from build123d import *

# Parameters (mm, degrees)
SKETCH_1_W          = 24
SKETCH_1_H          = 12
EXTRUDE_1_DEPTH     = 12
SKETCH_2_R          = 1
EXTRUDE_2_DEPTH     = 1.8
SKETCH_3_W          = 24
SKETCH_3_H          = 12
EXTRUDE_3_DEPTH     = 4
EXTRUDE_4_DEPTH     = 4
SKETCH_5_R          = 2
EXTRUDE_5_DEPTH     = 3.5
EXTRUDE_6_DEPTH     = 3
CUT_EXTRUDE_1_DEPTH = 12


with BuildPart() as part:
    # Эскиз1 → Бобышка-Вытянуть1 (new body)
    with BuildSketch(Plane.XY):
        Rectangle(SKETCH_1_W, SKETCH_1_H)
    extrude(amount=EXTRUDE_1_DEPTH)

    # Эскиз2 → Бобышка-Вытянуть2 (add)
    with BuildSketch(Plane(origin=(0, 0, 0), x_dir=(-1, 0, 0), z_dir=(0, 0, -1))):
        with BuildLine():
            Line((12, 6), (15, 6))
            ThreePointArc((15, 6), (15.707106781, 5.707106781), (16, 5))
            Line((16, 5), (16, -5))
            ThreePointArc((16, -5), (15.707106781, -5.707106781), (15, -6))
            Line((15, -6), (12, -6))
            Line((12, -6), (-12, -6))
            Line((-12, -6), (-15, -6))
            ThreePointArc((-15, -6), (-15.707106781, -5.707106781), (-16, -5))
            Line((-16, -5), (-16, 5))
            ThreePointArc((-16, 5), (-15.707106781, 5.707106781), (-15, 6))
            Line((-15, 6), (-12, 6))
            Line((-12, 6), (12, 6))
        make_face()
        with Locations((14, 0)):
            Circle(SKETCH_2_R, mode=Mode.SUBTRACT)
        with Locations((-14, 0)):
            Circle(SKETCH_2_R, mode=Mode.SUBTRACT)
    extrude(amount=EXTRUDE_2_DEPTH)

    # Эскиз3 → Бобышка-Вытянуть3 (add)
    with BuildSketch(Plane(origin=(0, 0, -1.8), x_dir=(-1, 0, 0), z_dir=(0, 0, -1))):
        Rectangle(SKETCH_3_W, SKETCH_3_H)
    extrude(amount=EXTRUDE_3_DEPTH)

    # Эскиз4 → Бобышка-Вытянуть4 (add)
    with BuildSketch(Plane(origin=(0, 0, -5.8), x_dir=(-1, 0, 0), z_dir=(0, 0, -1))):
        with BuildLine():
            ThreePointArc((0.75, 2.90473751), (12, 0), (0.75, -2.90473751))
            ThreePointArc((0.75, -2.90473751), (-3, 0), (0.75, 2.90473751))
        make_face()
    extrude(amount=EXTRUDE_4_DEPTH)

    # Эскиз5 → Бобышка-Вытянуть5 (add)
    with BuildSketch(Plane(origin=(0, 0, -9.8), x_dir=(-1, 0, 0), z_dir=(0, 0, -1))):
        with Locations((6, 0)):
            Circle(SKETCH_5_R)
    extrude(amount=EXTRUDE_5_DEPTH)

    # Эскиз6 → Бобышка-Вытянуть6 (add)
    with BuildSketch(Plane.XY.offset(12)):
        Polygon((12, -6), (12, 6), (-10, 6), (-10, 4), (-12, 4), (-12, -4), (-10, -4), (-10, -6), align=None)
    extrude(amount=EXTRUDE_6_DEPTH)

    # Эскиз8 → Вырез-Вытянуть1 (cut)
    with BuildSketch(Plane(origin=(0, 6, 0), x_dir=(1, 0, 0), z_dir=(0, 1, 0))):
        Polygon((-7, -15), (-12, -12), (-12, -15), align=None)
    extrude(amount=-CUT_EXTRUDE_1_DEPTH, mode=Mode.SUBTRACT)


solid = part.part
Verification items for the finished model (mm, model axes). A direction names the side the tool comes from. Round coordinates to 2 decimals unless told otherwise and drop trailing zeros. Order: outer loops, then holes, each group sorted by start corner. A loop starts at its lowest first (then second) coordinate and runs counter-clockwise, first axis right, second up. Notation, with made-up numbers: (61.5, -6) -> (72.5, -6) arc R16 ccw to (72.5, -1) -> close; hole circle Ø1 at (78, -33.75). An arc over 180 degrees is marked (long way). Put each result on its own line as item: value.
1) Section check C-C (z = -10.25). Record the cut outline in (x, y).
Final values:
outline: circle Ø4 at (-6, 0)
2) Section check D-D (z = 9). Record the cut outline in (x, y).
Final values:
outline: (-12, -6) -> (12, -6) -> (12, 6) -> (-12, 6) -> close
3) Set-up check for faces 1 (the flat face through (-3, 0, -9.8)), 2 (the flat face through (-10, 5, 13)), 3 (the flat face through (15.3, 0.1, -1.8)): record each of +Z, -Z, +X, -X, +Y, -Y from which the full face is reachable in a straight line by a thin tool's end or side.
Final values:
face 1: -Z
face 2: +Z, -X, +Y
face 3: -Z, +X, +Y, -Y
4) Material ranges on line 1 (Y direction, x = 14, z = -0.75); line 2 (Z direction, x = -10.5, y = -4.75); line 3 (X direction, y = 5.25, z = -2), recorded low to high.
Final values:
line 1: y = -6 to -1, 1 to 6
line 2: z = -5.8 to 12
line 3: x = -12 to 12
5) Depth check by flat-ended pin: pin 1 (1 mm diameter, centred on x = -11, y = 5.5, fed in from +Z); pin 2 (1.2 mm diameter, centred on x = -14, y = -0.5, fed in from +Z); pin 3 (1.2 mm diameter, centred on x = -14, y = 0, fed in from -Z); pin 4 (2 mm diameter, centred on y = 0, z = -4, fed in from -X). Enter the tip coordinate at first touch or a pass-through.
Final values:
pin 1: stops at z = 12
pin 2: stops at z = 0
pin 3: passes through
pin 4: stops at x = -12
6) Section check A-A (x = 14). Record the cut outline in (y, z), then the cut area to 3 significant figures.
Final values:
outline: (-6, -1.8) -> (-1, -1.8) -> (-1, 0) -> (-6, 0) -> close; (1, -1.8) -> (6, -1.8) -> (6, 0) -> (1, 0) -> close
area: 18.0 mm^2
7) Section check B-B (x = 0). Record the cut outline in (y, z).
Final values:
outline: (-6, -5.8) -> (-3, -5.8) -> (-3, -9.8) -> (3, -9.8) -> (3, -5.8) -> (6, -5.8) -> (6, 15) -> (-6, 15) -> close
